Check sheet for the modelled part. Datum: model origin and axes. Units: mm. Coordinates: 2 decimals unless noted, no trailing zeros. Loops run counter-clockwise (first coordinate to the right, second up) from the corner with the lowest first, then second, coordinate; pieces in that order, holes last. Notation, with made-up numbers: M 26.25,36.5 L 42.25,36.5 A29 ccw 42.25,67.5 Z; hole C 58,-26 d7. An arc over 180 degrees is marked long. Write each question's results on one line, items separated by ' | '. Start each with the question number.
from build123d import *

# Parameters (mm, degrees)
BOSS_EXTRUDE1_DEPTH                   = 3
M3_CLEARANCE_HOLE1_D                  = 3.2
M3_CLEARANCE_HOLE1_CSINK_D            = 3.25
M3_CLEARANCE_HOLE1_CSINK_ANGLE        = 90
FILLET1_R                             = 10
FILLET2_R                             = 3
TAP_DRILL_FOR_M3X0_5_TAP1_D           = 2.5
TAP_DRILL_FOR_M3X0_5_TAP1_CSINK_D     = 2.55
TAP_DRILL_FOR_M3X0_5_TAP1_CSINK_ANGLE = 90


with BuildPart() as part:
    # Sketch1 → Boss-Extrude1 (new body)
    with BuildSketch(Plane(origin=(0, 0, 0), x_dir=(1, 0, 0), z_dir=(0, 1, 0))):
        Polygon((0, 0), (194, 0), (194, -6.2), (221, -6.2), (221, 26.2), (221, 32), (0, 32), (0, 26.2), align=None)
    extrude(amount=BOSS_EXTRUDE1_DEPTH)

    # M3 Clearance Hole1 (through all)
    with Locations(Plane(origin=(0, 3, 0), x_dir=(1, 0, 0), z_dir=(0, 1, 0))):
        with Locations((197.5, 20), (217.5, 0), (217.5, 20), (197.5, 0)):
            CounterSinkHole(M3_CLEARANCE_HOLE1_D / 2, M3_CLEARANCE_HOLE1_CSINK_D / 2, counter_sink_angle=M3_CLEARANCE_HOLE1_CSINK_ANGLE)

    # Fillet1
    # the kernel refuses this fillet: 10 mm, written as the material it adds along each edge
    with BuildSketch(Plane(origin=(194, 0, 0), x_dir=(-1, 0, 0), z_dir=(0, 1, 0))) as fillet1_piece_1:
        with BuildLine():
            CenterArc((9.249864864, 10), FILLET1_R, 202.333682658, 67.666317342)
            Line((0, 6.2), (-0.184997297, 6.124))
            ThreePointArc((-0.184997297, 6.124), (-0.2, 3.1), (-0.2, 0))
            Line((-0.2, 0), (0, -0.2))
            Line((0, -0.2), (9.249864864, -0.2))
            Line((9.249864864, -0.2), (9.249864864, 0))
        make_face()
    extrude(amount=3)

    # Fillet2
    fillet2_edges = [part.edges().sort_by_distance(p)[0] for p in [
        (221, 1.5, -32),
        (221, 1.5, 6.2),
        (194, 1.5, 6.2),
    ]]
    fillet(fillet2_edges, radius=FILLET2_R)

    # Mirror1: part across plane


with BuildPart() as part_1:
    add(part.part)
    add(part.part.mirror(Plane(origin=(0, 3, -32), x_dir=(0, 0, 1), z_dir=(1, 0, 0))))

    # Tap Drill for M3x0.5 Tap1 (through all)
    with Locations(Plane(origin=(0, 3, 0), x_dir=(1, 0, 0), z_dir=(0, 1, 0))):
        with Locations((-170, 10), (-150, 10), (-130, 10), (-110, 10), (-90, 10), (-70, 10), (-50, 10), (-30, 10), (-10, 10), (10, 10), (30, 10), (50, 10), (70, 10), (170, 10), (150, 10), (130, 10), (110, 10), (90, 10)):
            CounterSinkHole(TAP_DRILL_FOR_M3X0_5_TAP1_D / 2, TAP_DRILL_FOR_M3X0_5_TAP1_CSINK_D / 2, counter_sink_angle=TAP_DRILL_FOR_M3X0_5_TAP1_CSINK_ANGLE)


solid = part_1.part
1) Gauge pin test, flat end, axial feed: P1, Ø3, axis at x = -197.5, z = 0, coming from the +Y side. Record the tip position at first contact, or that the pin passes through.
2) Section check B-B (x = 95). Enter the section's corners in (y, z).
3) Section check A-A (y = 2.5). Give the number of separate pieces and of enclosed holes in the cut face, then the cut area to 3 significant figures.
4) Thickness scan on probe 1 along Z at (x, y) = (217.5, 1.7); probe 2 along Z at (x, y) = (-130, 0.6); probe 3 along X at (y, z) = (2.05, -29.5). Record the ranges inside material, lowest first.
Return value:
1) P1: passes through
2) outline: M 0,-32 L 3,-32 L 3,0 L 0,0 Z
3) separate pieces: 1 | enclosed holes: 26 | area: 14,300 mm2
4) probe 1: z = -32 to -21.6, -18.4 to -1.6, 1.6 to 6.2 | probe 2: z = -32 to -11.25, -8.75 to 0 | probe 3: x = -220.96 to 220.96
